Can you work these out from the model? Positions are in its coordinate system, mm. A direction names the side the tool comes from. Round coordinates to 2 decimals unless told otherwise and drop trailing zeros. Order: outer loops, then holes, each group sorted by start corner. A loop starts at its lowest first (then second) coordinate and runs counter-clockwise, first axis right, second up. Notation, with made-up numbers: (34, -24.75) -> (67, -24.75) arc R34 cw to (67, 11.25) -> close; hole circle Ø1 at (18, -23). An arc over 180 degrees is marked (long way). Use a Markdown table: item, result. Add a question column.
Q1. For faces 5 (the face through (88, 3, -177.8)), 6 (the face through (76, 3, -6.35)), which set-ups out of +Z, -Z, +X, -X, +Y, -Y let a thin tool reach every point of the face, with its end or its side?
Q2. I need wall thicknesses on line 1 along Z through (x, y) = (34, 2); line 2 along X through (y, z) = (1.9, -5.16); line 3 along X through (y, z) = (2.95, -51.32) (3 decimals). Which ranges of each line are inside material? Lowest first, please. Write a range as [from, to].
Q3. If we section it at A-A on z = -76.2: List the corners of the cut face in (x, y) for me, plus the area to 3 significant figures.
Q4. We'd pull the mould along X, two halves only. Please class faces 1 (the face through (0, 3, -88)), 2 (the face through (84.214, 3, -3)), 3 (the face through (177.8, 3, -88)), 4 (the face through (88, 5.994, -90)): +X half, -X half, draft (parallel to the pull), parting line (faces both ways), or undercut.
Q5. If we section it at B-B on x = 79.5: List the corners of the cut face in (y, z) for me.
Q6. I'm going to push a flat-ended pin straight in: pin 1 Ø3 at (x, y) = (78.5, 4) entering from +Z. Where does the tip first touch, or does it pass through?
```python
from build123d import *

# Parameters (mm, degrees)
SKETCH1_W               = 177.8
SKETCH1_H               = 177.8
BOSS_EXTRUDE1_DEPTH     = 5.9944
CUT_EXTRUDE1_DEPTH      = 252.51861329
CUT_EXTRUDE1_DEPTH_BACK = 5.9944
SKETCH5_R               = 1.6
CUT_EXTRUDE2_DEPTH      = 252.51861329
CUT_EXTRUDE2_DEPTH_BACK = 252.51861329
SKETCH6_W               = 15.24
SKETCH6_H               = 6.35
CUT_EXTRUDE3_DEPTH      = 252.51861329
CUT_EXTRUDE3_DEPTH_BACK = 252.51861329
SKETCH7_R               = 1.6
CUT_EXTRUDE4_DEPTH      = 252.51861329
CUT_EXTRUDE4_DEPTH_BACK = 252.51861329
SKETCH8_R               = 6.35
CUT_EXTRUDE5_DEPTH      = 252.51861329
CUT_EXTRUDE5_DEPTH_BACK = 252.51861329
SKETCH9_R               = 1.363261963
SKETCH9_R_2             = 1.386126721


with BuildPart() as part:
    # Sketch1 → Boss-Extrude1 (new body)
    with BuildSketch(Plane(origin=(0, 0, 0), x_dir=(1, 0, 0), z_dir=(0, 1, 0))):
        with Locations((88.9, 88.9)):
            Rectangle(SKETCH1_W, SKETCH1_H)
    extrude(amount=BOSS_EXTRUDE1_DEPTH)

    # Sketch5 → Cut-Extrude1 (cut, two sides: drawn at the far end of the back side and taken through both)
    with BuildSketch(Plane.XZ.offset(-CUT_EXTRUDE1_DEPTH_BACK)):
        with Locations(Location((163, -22.25, 0), (0, 0, 270))):
            Circle(SKETCH5_R)
        with Locations(Location((163, -53.45, 0), (0, 0, 270))):
            Circle(SKETCH5_R)
        with Locations(Location((143.8, -22.25, 0), (0, 0, 270))):
            Circle(SKETCH5_R)
        with Locations(Location((143.8, -53.45, 0), (0, 0, 270))):
            Circle(SKETCH5_R)
        with Locations(Location((14.8, -22.25, 0), (0, 0, 270))):
            Circle(SKETCH5_R)
        with Locations(Location((14.8, -53.45, 0), (0, 0, 270))):
            Circle(SKETCH5_R)
        with Locations(Location((40.4, -130.7, 0), (0, 0, 270))):
            Circle(SKETCH5_R)
        with Locations(Location((14.8, -130.7, 0), (0, 0, 270))):
            Circle(SKETCH5_R)
        with Locations(Location((14.8, -161.9, 0), (0, 0, 270))):
            Circle(SKETCH5_R)
        with Locations(Location((40.4, -161.9, 0), (0, 0, 270))):
            Circle(SKETCH5_R)
        with Locations(Location((163, -130.7, 0), (0, 0, 270))):
            Circle(SKETCH5_R)
        with Locations(Location((163, -161.9, 0), (0, 0, 270))):
            Circle(SKETCH5_R)
        with Locations(Location((137.4, -130.7, 0), (0, 0, 270))):
            Circle(SKETCH5_R)
        with Locations(Location((137.4, -161.9, 0), (0, 0, 270))):
            Circle(SKETCH5_R)
        with Locations(Location((34, -22.25, 0), (0, 0, 270))):
            Circle(SKETCH5_R)
        with Locations(Location((34, -53.45, 0), (0, 0, 270))):
            Circle(SKETCH5_R)
    extrude(amount=CUT_EXTRUDE1_DEPTH + CUT_EXTRUDE1_DEPTH_BACK, mode=Mode.SUBTRACT)

    # Sketch6 → Cut-Extrude2 (cut, two sides: drawn at the far end of the back side and taken through both)
    with BuildSketch(Plane(origin=(0, 5.9944, 0), x_dir=(1, 0, 0), z_dir=(0, 1, 0)).offset(-CUT_EXTRUDE2_DEPTH_BACK)):
        with Locations((76.5936, 3.175)):
            Rectangle(SKETCH6_W, SKETCH6_H)
    extrude(amount=CUT_EXTRUDE2_DEPTH + CUT_EXTRUDE2_DEPTH_BACK, mode=Mode.SUBTRACT)

    # Sketch7 → Cut-Extrude3 (cut, two sides: drawn at the far end of the back side and taken through both)
    with BuildSketch(Plane(origin=(0, 5.9944, 0), x_dir=(1, 0, 0), z_dir=(0, 1, 0)).offset(-CUT_EXTRUDE3_DEPTH_BACK)):
        with Locations(Location((55.9736, 51.32, 0), (0, 0, 270))):
            Circle(SKETCH7_R)
        with Locations(Location((102.855, 51.32, 0), (0, 0, 270))):
            Circle(SKETCH7_R)
        with Locations(Location((122.855, 20.35, 0), (0, 0, 270))):
            Circle(SKETCH7_R)
        with Locations(Location((55.9736, 27, 0), (0, 0, 270))):
            Circle(SKETCH7_R)
    extrude(amount=CUT_EXTRUDE3_DEPTH + CUT_EXTRUDE3_DEPTH_BACK, mode=Mode.SUBTRACT)

    # Sketch8 → Cut-Extrude4 (cut, two sides: drawn at the far end of the back side and taken through both)
    with BuildSketch(Plane(origin=(0, 5.9944, 0), x_dir=(1, 0, 0), z_dir=(0, 1, 0)).offset(-CUT_EXTRUDE4_DEPTH_BACK)):
        with Locations(Location((88.9, 76.2, 0), (0, 0, 270))):
            Circle(SKETCH8_R)
    extrude(amount=CUT_EXTRUDE4_DEPTH + CUT_EXTRUDE4_DEPTH_BACK, mode=Mode.SUBTRACT)

    # Sketch9 → Cut-Extrude5 (cut, two sides: drawn at the far end of the back side and taken through both)
    with BuildSketch(Plane(origin=(0, 0, 0), x_dir=(-1, 0, 0), z_dir=(0, -1, 0)).offset(-CUT_EXTRUDE5_DEPTH_BACK)):
        with Locations(Location((-37.15, 5.16, 0), (0, 0, 90))):
            Circle(SKETCH9_R)
        with Locations(Location((-135.15, 5.16, 0), (0, 0, 90))):
            Circle(SKETCH9_R_2)
    extrude(amount=CUT_EXTRUDE5_DEPTH + CUT_EXTRUDE5_DEPTH_BACK, mode=Mode.SUBTRACT)


solid = part.part
```
Answer below:
| question | item | result |
|---|---|---|
| 1 | face 5 | -Z, +X, -X, +Y, -Y |
| 1 | face 6 | +Z, +Y, -Y |
| 2 | line 1 | [-177.8, -55.05], [-51.85, -23.85], [-20.65, 0] |
| 2 | line 2 | [0, 35.79], [38.51, 68.97], [84.21, 133.76], [136.54, 177.8] |
| 2 | line 3 | [0, 54.374], [57.574, 101.255], [104.455, 177.8] |
| 3 | outline | (0, 0) -> (82.55, 0) -> (82.55, 5.99) -> (0, 5.99) -> close; (95.25, 0) -> (177.8, 0) -> (177.8, 5.99) -> (95.25, 5.99) -> close |
| 3 | area | 990 mm² |
| 4 | face 1 | -X half |
| 4 | face 2 | undercut |
| 4 | face 3 | +X half |
| 4 | face 4 | draft |
| 5 | outline | (0, -177.8) -> (5.99, -177.8) -> (5.99, -6.35) -> (0, -6.35) -> close |
| 6 | pin 1 | z = -6.35 |
